```python
from build123d import *

# Parameters (mm, degrees)
BOSS_EXTRUDE1_DEPTH = 65
SHELL1_T            = -5
CUT_EXTRUDE1_DEPTH  = 373.86056375
SKETCH4_W           = 245
SKETCH4_H           = 53.856180832
CUT_EXTRUDE2_DEPTH  = 3.75


# Read off the part's stored shape, not the designer's step: Boss-Extrude1
with BuildPart() as part:
    # Boss-Extrude1 outline → Boss-Extrude1 (new body)
    with BuildSketch(Plane(origin=(0, 0, 0), x_dir=(0, 1, 0), z_dir=(0, 0, 1))):
        with BuildLine():
            ThreePointArc((105, -162.5), (158.033008589, -140.533008589), (180, -87.5))
            Line((180, -87.5), (180, 152.5))
            ThreePointArc((180, 152.5), (177.071067812, 159.571067812), (170, 162.5))
            Line((170, 162.5), (-170, 162.5))
            ThreePointArc((-170, 162.5), (-177.071067812, 159.571067812), (-180, 152.5))
            Line((-180, 152.5), (-180, -87.5))
            ThreePointArc((-180, -87.5), (-158.033008589, -140.533008589), (-105, -162.5))
            Line((-105, -162.5), (105, -162.5))
        make_face()
    extrude(amount=BOSS_EXTRUDE1_DEPTH)

    # Shell1
    shell1_openings = [part.faces().sort_by_distance(p)[0] for p in [
        (-3.011930619, 0, 65),
    ]]
    offset(amount=SHELL1_T, openings=shell1_openings, kind=Kind.INTERSECTION)

    # Sketch3 → Cut-Extrude1 (cut, through all)
    with BuildSketch(Plane.YZ.offset(-157.5)):
        with BuildLine():
            Line((-148.652392821, 16.9228), (-141.347607179, 16.9228))
            ThreePointArc((-141.347607179, 16.9228), (-145, 33.8646), (-148.652392821, 16.9228))
        make_face()
        with BuildLine():
            Line((-125.319059488, 35.778980832), (-118.014273846, 35.778980832))
            ThreePointArc((-118.014273846, 35.778980832), (-121.666666667, 52.720780832), (-125.319059488, 35.778980832))
        make_face()
        with BuildLine():
            Line((-78.652392821, 35.778980832), (-71.347607179, 35.778980832))
            ThreePointArc((-71.347607179, 35.778980832), (-75, 52.720780832), (-78.652392821, 35.778980832))
        make_face()
        with BuildLine():
            Line((-101.985726154, 16.9228), (-94.680940512, 16.9228))
            ThreePointArc((-94.680940512, 16.9228), (-98.333333333, 33.8646), (-101.985726154, 16.9228))
        make_face()
        with BuildLine():
            Line((-31.985726154, 35.778980832), (-24.680940512, 35.778980832))
            ThreePointArc((-24.680940512, 35.778980832), (-28.333333333, 52.720780832), (-31.985726154, 35.778980832))
        make_face()
        with BuildLine():
            Line((-55.319059488, 16.9228), (-48.014273846, 16.9228))
            ThreePointArc((-48.014273846, 16.9228), (-51.666666667, 33.8646), (-55.319059488, 16.9228))
        make_face()
        with BuildLine():
            Line((14.680940512, 35.778980832), (21.985726154, 35.778980832))
            ThreePointArc((21.985726154, 35.778980832), (18.333333333, 52.720780832), (14.680940512, 35.778980832))
        make_face()
        with BuildLine():
            Line((-8.652392821, 16.9228), (-1.347607179, 16.9228))
            ThreePointArc((-1.347607179, 16.9228), (-5, 33.8646), (-8.652392821, 16.9228))
        make_face()
        with BuildLine():
            Line((61.347607179, 35.778980832), (68.652392821, 35.778980832))
            ThreePointArc((68.652392821, 35.778980832), (65, 52.720780832), (61.347607179, 35.778980832))
        make_face()
        with BuildLine():
            Line((38.014273846, 16.9228), (45.319059488, 16.9228))
            ThreePointArc((45.319059488, 16.9228), (41.666666667, 33.8646), (38.014273846, 16.9228))
        make_face()
    extrude(amount=-CUT_EXTRUDE1_DEPTH, mode=Mode.SUBTRACT)

    # Sketch4 → Cut-Extrude2 (cut)
    with BuildSketch(Plane.YZ.offset(-157.5)):
        with Locations((-40, 34.428090416)):
            Rectangle(SKETCH4_W, SKETCH4_H)
    extrude(amount=-CUT_EXTRUDE2_DEPTH, mode=Mode.SUBTRACT)


solid = part.part
```
Work out the finished part from the listing and answer in its coordinate system (mm). A direction names the side the tool comes from. Coordinates: 2 decimals unless noted, no trailing zeros. Write each loop counter-clockwise with the first axis right and the second up, starting at its lowest first coordinate (ties: lowest second). Pieces come first, ordered by that corner, then holes.
Q1. Which of the six approach directions +Z, -Z, +X, -X, +Y, -Y give full straight-line access (tool end or side, diameter ignored) to faces 5 (the face through (-2, -2, 5)), 6 (the face through (141.11, 157.45, 32.04)), 7 (the face through (-161.87, -51.33, 33.86))?
Q2. Find the intervals of material crossed by line 1 (X direction, y = 95, z = 7); line 2 (X direction, y = -45, z = 59.5); line 3 (Y direction, x = -29, z = 37), in increasing order.
Q3. Each of these flat-tipped pins is pushed along its axis until it touches: pin 1 Ø10 at (x, y) = (100, 43) entering from -Z; pin 2 Ø14 at (y, z) = (-51.67, 25) entering from -X; pin 3 Ø1.1 at (x, z) = (-160, 30) entering from -Y; pin 4 Ø4 at (y, z) = (112.5, 48) entering from +X. Where does it stop, or does it pass through?
Q4. A cutting plane is placed at A-A, the plane y = 90.5. Give the vertices of the cut face in (x, z), then the cut area to 4 significant figures.
Q5. A cutting plane is placed at C-C, the plane z = 42. State how many separate pieces and enclosed holes the cut face has, then the cut area to 3 significant figures.
Q6. A cutting plane is placed at B-B, the plane x = -33.5. Give the vertices of the cut face in (y, z), then the cut area to 3 significant figures.
Q7. Determine the mould class of faces 1 (the face through (-161.25, -42, 35)), 2 (the face through (139.95, -158.61, 32.04)), 3 (the face through (-162.5, 2, 32)), 4 (the face through (-161.87, -4.66, 33.86)) for opening direction X: released by +X, released by -X, zero draft, split by the parting line, or undercut.
Findings below:
1. face 5: +Z
1. face 6: +Z, -Z, +X, +Y
1. face 7: -X
2. line 1: x = -162.5 to -157.5, 157.5 to 162.5
2. line 2: x = -162.5 to -161.25, 157.5 to 162.5
2. line 3: y = -180 to -175, 175 to 180
3. pin 1: stops at z = 0
3. pin 2: stops at x = 157.5
3. pin 3: stops at y = -177.19
3. pin 4: stops at x = 162.3
4. outline: (-162.5, 0) - (162.5, 0) - (162.5, 65) - (157.5, 65) - (157.5, 5) - (-157.5, 5) - (-157.5, 65) - (-162.5, 65) - close
4. area: 2,225 mm2
5. separate pieces: 5
5. enclosed holes: 0
5. area: 5,380 mm2
6. outline: (-180, 0) - (180, 0) - (180, 65) - (175, 65) - (175, 5) - (-175, 5) - (-175, 65) - (-180, 65) - close
6. area: 2,400 mm2
7. face 1: undercut
7. face 2: released by +X
7. face 3: released by -X
7. face 4: zero draft
